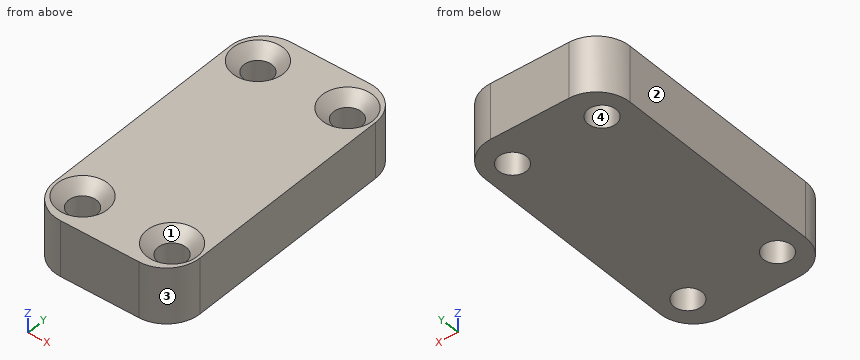
from build123d import *

# Parameters (mm, degrees)
F0_W     = 13
F0_H     = 25
F0_R     = 1.25
F1_DEPTH = 5
F2_R     = 3
F3_SIZE  = 1


with BuildPart() as f1:
    # F0 (on Top) → F1 (new body)
    with BuildSketch(Plane.XY):
        Rectangle(F0_W, F0_H)
        with Locations((-4, -9.5)):
            Circle(F0_R, mode=Mode.SUBTRACT)
        with Locations((4, -9.5)):
            Circle(F0_R, mode=Mode.SUBTRACT)
        with Locations((-4, 9.5)):
            Circle(F0_R, mode=Mode.SUBTRACT)
        with Locations((4, 9.5)):
            Circle(F0_R, mode=Mode.SUBTRACT)
    extrude(amount=F1_DEPTH)

    # F2
    f2_edges = [f1.edges().sort_by_distance(p)[0] for p in [
        (-6.5, -12.5, 2.5),
        (6.5, -12.5, 2.5),
        (6.5, 12.5, 2.5),
        (-6.5, 12.5, 2.5),
    ]]
    fillet(f2_edges, radius=F2_R)

    # F3
    f3_edges = [f1.edges().sort_by_distance(p)[0] for p in [
        (-5.25, 9.5, 5),
        (2.75, 9.5, 5),
        (2.75, -9.5, 5),
        (-5.25, -9.5, 5),
    ]]
    chamfer(f3_edges, length=F3_SIZE)


solid = f1.part
Source: CAD feature listing. Evaluate the final solid. Frame: model axes, mm. Face numbers are marked on the shaded views. Round coordinates to 2 decimals unless told otherwise and drop trailing zeros. Loops run counter-clockwise (first coordinate to the right, second up) from the corner with the lowest first, then second, coordinate; pieces in that order, holes last. Notation, with made-up numbers: (65.25, -27.75) - (84.25, -27.75) arc R8 ccw to (84.25, -14.75) - close; hole circle Ø11 at (59, -22.5). An arc over 180 degrees is marked (long way). Write item = value, one per line. Start each with the question number.
Item 1: Mould query, pull axis Y, two halves, no side actions, for the marked faces 1, 2, 3 and 4. Classes: released by +Y, released by -Y, zero draft, split by the parting line, or undercut.
Item 2: Section query A-A on z = 4.5. Output: boundary loops of the cut face in (x, y).
Item 3: Section query D-D on x = 4.5. Count the separate pieces of the cut face and the enclosed holes in it, plus the area to 3 significant figures.
Item 4: Section query C-C on z = 2.65. Output: boundary loops of the cut face in (x, y).
Item 5: Section query B-B on x = -4. Output: boundary loops of the cut face in (y, z).
Item 6: First-contact query: pin 1 Ø1.5 at (x, y) = (4, -9.5) entering from +Z. Flat tip, straight axial feed; report the tip coordinate or a pass-through.
Item 7: Material intervals for line 1 (Y direction, x = -4, z = 2.1); line 2 (Y direction, x = -5, z = 0.65); line 3 (X direction, y = 10.5, z = 4.5), sorted ascending.
Results list:
q1.face_1 = undercut
q1.face_2 = zero draft
q1.face_3 = released by -Y
q1.face_4 = undercut
q2.outline = (-6.5, -9.5) arc R3 ccw to (-3.5, -12.5) - (3.5, -12.5) arc R3 ccw to (6.5, -9.5) - (6.5, 9.5) arc R3 ccw to (3.5, 12.5) - (-3.5, 12.5) arc R3 ccw to (-6.5, 9.5) - close; hole circle Ø3.5 at (-4, -9.5); hole circle Ø3.5 at (-4, 9.5); hole circle Ø3.5 at (4, -9.5); hole circle Ø3.5 at (4, 9.5)
q3.separate_pieces = 3
q3.enclosed_holes = 0
q3.area = 98.3 mm²
q4.outline = (-6.5, -9.5) arc R3 ccw to (-3.5, -12.5) - (3.5, -12.5) arc R3 ccw to (6.5, -9.5) - (6.5, 9.5) arc R3 ccw to (3.5, 12.5) - (-3.5, 12.5) arc R3 ccw to (-6.5, 9.5) - close; hole circle Ø2.5 at (-4, -9.5); hole circle Ø2.5 at (-4, 9.5); hole circle Ø2.5 at (4, -9.5); hole circle Ø2.5 at (4, 9.5)
q5.outline = (-12.46, 0) - (-10.75, 0) - (-10.75, 4) - (-11.75, 5) - (-12.46, 5) - close; (-8.25, 0) - (8.25, 0) - (8.25, 4) - (7.25, 5) - (-7.25, 5) - (-8.25, 4) - close; (10.75, 0) - (12.46, 0) - (12.46, 5) - (11.75, 5) - (10.75, 4) - close
q6.pin_1 = through
q7.line_1 = -12.46 to -10.75, -8.25 to 8.25, 10.75 to 12.46
q7.line_2 = -12.1 to -10.25, -8.75 to 8.75, 10.25 to 12.1
q7.line_3 = -6.33 to -5.44, -2.56 to 2.56, 5.44 to 6.33
